Can you work these out from the model? Positions are in its coordinate system, mm. A direction names the side the tool comes from. Give positions to 0.01 mm unless a question says otherwise; leave off trailing zeros. Loops run counter-clockwise (first coordinate to the right, second up) from the corner with the lowest first, then second, coordinate; pieces in that order, holes last.
from build123d import *

# Parameters (mm, degrees)
SKETCH1_R               = 15
BOSS_EXTRUDE1_DEPTH     = 10
SKETCH2_W               = 25
SKETCH2_H               = 30
SKETCH2_R               = 11.1
BOSS_EXTRUDE3_DEPTH     = 10
SKETCH6_R               = 1.5
CUT_EXTRUDE2_DEPTH      = 10
CUT_EXTRUDE3_START      = -10
SKETCH4_R               = 4
CUT_EXTRUDE3_DEPTH      = 6.5
SKETCH7_R               = 1.5
CUT_EXTRUDE4_DEPTH      = 14
CUT_EXTRUDE5_REACH      = 117.758
CUT_EXTRUDE5_END_RADIUS = 4
SKETCH8_R               = 1.5


with BuildPart() as part:
    # Sketch1 → Boss-Extrude1 (new body)
    with BuildSketch(Plane(origin=(0, 0, 0), x_dir=(1, 0, 0), z_dir=(0, 1, 0))):
        with BuildLine():
            Line((-110, 15), (-110, -15))
            Line((-110, -15), (95, -15))
            ThreePointArc((95, -15), (80, 0), (95, 15))
            Line((95, 15), (-110, 15))
        make_face()
        with Locations((95, 0)):
            Circle(SKETCH1_R)
    extrude(amount=BOSS_EXTRUDE1_DEPTH)

    # Sketch2 → Boss-Extrude3 (add)
    with BuildSketch(Plane(origin=(0, 10, 0), x_dir=(1, 0, 0), z_dir=(0, 1, 0))):
        with Locations((-97.5, 0)):
            Rectangle(SKETCH2_W, SKETCH2_H)
        with Locations(Location((-97.5, 0, 0), (0, 0, 270))):
            Circle(SKETCH2_R, mode=Mode.SUBTRACT)
    extrude(amount=BOSS_EXTRUDE3_DEPTH)

    # Sketch6 → Cut-Extrude2 (cut)
    with BuildSketch(Plane.XY.offset(15)):
        with Locations((-97.5, 15)):
            Circle(SKETCH6_R)
    extrude(amount=-CUT_EXTRUDE2_DEPTH, mode=Mode.SUBTRACT)

    # Sketch4 → Cut-Extrude3 (cut)
    with BuildSketch(Plane(origin=(0, 10, 0), x_dir=(1, 0, 0), z_dir=(0, 1, 0)).offset(CUT_EXTRUDE3_START)):
        with Locations(Location((90, 0, 0), (0, 0, 90))):
            Circle(SKETCH4_R)
    extrude(amount=CUT_EXTRUDE3_DEPTH, mode=Mode.SUBTRACT)

    # Sketch7 → Cut-Extrude4 (cut)
    with BuildSketch(Plane(origin=(0, 6.5, 0), x_dir=(-1, 0, 0), z_dir=(0, -1, 0))):
        with Locations(Location((-90, 0, 0), (0, 0, 90))):
            Circle(SKETCH7_R)
    extrude(amount=-CUT_EXTRUDE4_DEPTH, mode=Mode.SUBTRACT)

    # Cut-Extrude5: up to this cylinder (the profile starts outside it)
    cut_extrude5_end = Plane(origin=(90, 3, 0), z_dir=(0, -1, 0)) * Cylinder(CUT_EXTRUDE5_END_RADIUS, 244.516, mode=Mode.PRIVATE)
    # Sketch8 → Cut-Extrude5 (cut, up to the surface)
    with BuildSketch(Plane(origin=(0, 0, -15), x_dir=(-1, 0, 0), z_dir=(0, 0, -1)), mode=Mode.PRIVATE) as cut_extrude5_sk1:
        with Locations((-90, 3)):
            Circle(SKETCH8_R)
    cut_extrude5_tool1 = extrude(cut_extrude5_sk1.sketch, amount=-CUT_EXTRUDE5_REACH, mode=Mode.PRIVATE) - cut_extrude5_end
    add(cut_extrude5_tool1.solids().sort_by_distance((90, 3, -15))[0], mode=Mode.SUBTRACT)


solid = part.part
(1) Will these pins go through, and if not, where does the flat tip stop? P1, Ø8, axis at x = -9.5, z = -7.5, coming from the +Y side; P2, Ø2.5, axis at x = 88, z = -1, coming from the -Y side; P3, Ø1.8, axis at x = 90, z = 0, coming from the +Y side; P4, Ø8, axis at y = 14.5, z = 6, coming from the +X side.
Returned:
P1: stops at y = 10
P2: stops at y = 6.5
P3: passes through
P4: stops at x = -85
(2) Which directions (+Z, -Z, +X, -X, +Y, -Y) give clear straight access to the entire face, cutting with the end or side of a thin tool? Please do faces 1 (the flat face through (11, 10, 0)), 2 (the flat face through (92, 6.5, 0)), 3 (the flat face through (-98, 10, 0)).
Returned:
face 1: +Z, -Z, +X, +Y
face 2: -Y
face 3: +Y
(3) Thinking about a two-plate mould opening in Z: for faces 4 (the flat face through (-9, 5, 15)), 5 (the cylindrical face through (92.4, 3.2, 3.2)), 6 (the cylindrical face through (110, 5, 0)), which applies, pulls with the +Z half, pulls with the -Z half, needs draft (parallel to the pull), parting line crosses it, or undercut?
Returned:
face 4: pulls with the +Z half
face 5: undercut
face 6: parting line crosses it
(4) Please list where these lines run through material, in increasing order: probe 1 along X at (y, z) = (15, 13.1); probe 2 along Z at (x, y) = (90, 8); probe 3 along X at (y, z) = (8.1, 0).
Returned:
probe 1: x = -110 to -99, -96 to -85
probe 2: z = -15 to -1.5, 1.5 to 15
probe 3: x = -110 to 88.5, 91.5 to 110
(5) Suppose I cut it at A-A on x = 68. List the corners of the cut face in (y, z) for me, plus the area to 3 significant figures.
Returned:
outline: (0, -15) - (10, -15) - (10, 15) - (0, 15) - close
area: 300 mm2
